Solid Edge part; units mm, degrees
sketch "Sketch1" plane through (0, 0, 0) normal (0, -1, 0) x (1, 0, 0)
  line L0 (7.5, 0) -> (3.8603, 10)
  line L1 (3.8603, 10) -> (0, 10)
  line L2 (-3.8603, 10) -> (0, 10)
  line L3 (-7.5, 0) -> (-3.8603, 10)
  line L4 (0, 0) -> (-7.5, 0)
  line L5 (0, 0) -> (7.5, 0)
  circle A0 centre (0, 5) radius 1.5
extrude "Protrusion1" add sketch "Sketch1" against normal blind 10
Geometry check sheet. Reference: the model listing, model coordinates, mm. Give positions to 0.01 mm unless a question says otherwise; leave off trailing zeros. Order: outer loops, then holes, each group sorted by start corner. A loop starts at its lowest first (then second) coordinate and runs counter-clockwise, first axis right, second up.
1. Sectioned sample at A-A (x = 0). Record the boundary of the cut face in (y, z).
Completed:
outline: (0, 0) - (10, 0) - (10, 3.5) - (0, 3.5) - close; (0, 6.5) - (10, 6.5) - (10, 10) - (0, 10) - close
2. Sectioned sample at C-C (z = 5). Record the boundary of the cut face in (x, y).
Completed:
outline: (-5.68, 0) - (-1.5, 0) - (-1.5, 10) - (-5.68, 10) - close; (1.5, 0) - (5.68, 0) - (5.68, 10) - (1.5, 10) - close
3. Sectioned sample at D-D (z = 1). Record the boundary of the cut face in (x, y).
Completed:
outline: (-7.14, 0) - (7.14, 0) - (7.14, 10) - (-7.14, 10) - close
4. Scan lines: line 1 (Z direction, x = 0, y = 6.25); line 2 (X direction, y = 2, z = 5.75); line 3 (X direction, y = 2, z = 4.75). Record each from-to range of solid material in increasing order.
Completed:
line 1: z = 0 to 3.5, 6.5 to 10
line 2: x = -5.41 to -1.3, 1.3 to 5.41
line 3: x = -5.77 to -1.48, 1.48 to 5.77
5. Sectioned sample at B-B (y = 9.5). Record the boundary of the cut face in (x, z).
Completed:
outline: (-7.5, 0) - (7.5, 0) - (3.86, 10) - (-3.86, 10) - close; hole circle Ø3 at (0, 5)
6. Depth check by flat-ended pin: pin 1 (2 mm diameter, centred on x = -5, y = 4, fed in from -Z); pin 2 (1.5 mm diameter, centred on y = 1.5, z = 9, fed in from +X). Enter the tip coordinate at first touch or a pass-through.
Completed:
pin 1: stops at z = 0
pin 2: stops at x = 4.5
7. Draft check along Z on faces 1 (the face through (-1.5, 4.93, 5.07)), 2 (the face through (0, 0, 3)), 3 (the face through (0, 5, 10)). Enter one of: pulls with the +Z half, pulls with the -Z half, needs draft (parallel to the pull), parting line crosses it, or undercut.
Completed:
face 1: undercut
face 2: needs draft
face 3: pulls with the +Z half
